Verification items for the finished model (mm, model axes). A direction names the side the tool comes from. Round coordinates to 2 decimals unless told otherwise and drop trailing zeros. Write each loop counter-clockwise with the first axis right and the second up, starting at its lowest first coordinate (ties: lowest second). Pieces come first, ordered by that corner, then holes. Notation, with made-up numbers: M 89.5,-23 L 111.5,-23 A24 cw 111.5,5 Z; hole C 39.5,63.5 d3. An arc over 180 degrees is marked long. Answer in a Markdown table with one row per item. Add a question column.
1. Sectioned sample at C-C on z = 19. Record the cut outline in (x, y).
2. Go/stop test with flat-tipped pins: pin 1 Ø1 at (x, y) = (-9.5, -0.5) entering from +Z; pin 2 Ø10 at (y, z) = (-9.5, 12) entering from +X; pin 3 Ø12 at (y, z) = (6.5, 20.5) entering from -X; pin 4 Ø5 at (x, y) = (6, -0.5) entering from -Z. Record where each tip stops, or that it passes through.
3. Draft check along Y on faces 1 (the cylindrical face through (12.932, -5.362, 35.479)), 2 (the flat face through (3, -3, 63)), 3 (the flat face through (-10, 0, 53)). Enter one of: pulls with the +Y half, pulls with the -Y half, needs draft (parallel to the pull), parting line crosses it, or undercut.
4. Sectioned sample at D-D on y = -11. Record the cut outline in (x, z), plus the area to 3 significant figures.
5. Set-up check for faces 4 (the cylindrical face through (2.93, -13.18, 37.49)), 5 (the cylindrical face through (12.932, -5.362, 6.902)), 6 (the flat face through (0, 0, 0)), 7 (the cylindrical face through (3.233, -1.341, 63.986)), 8 (the flat face through (0, 0, 77)): record each of +Z, -Z, +X, -X, +Y, -Y from which the full face is reachable in a straight line by a thin tool's end or side.
6. Material ranges on probe 1 along Z at (x, y) = (-1.75, 11.5); probe 2 along Z at (x, y) = (0.5, -2.5); probe 3 along Y at (x, z) = (10, 55.5), recorded low to high.
7. Sectioned sample at A-A on x = 0. Record the cut outline in (y, z), plus the area to 4 significant figures.
8. Sectioned sample at B-B on y = 10. Record the cut outline in (x, z), plus the area to 3 significant figures.
```python
from build123d import *

# Parameters (mm, degrees)
SKETCH1_R           = 14
BOSS_EXTRUDE1_DEPTH = 63
SKETCH2_R           = 3.5
BOSS_EXTRUDE2_DEPTH = 2
SKETCH3_R           = 2
BOSS_EXTRUDE3_DEPTH = 12
SKETCH4_R           = 14.5
BOSS_EXTRUDE4_DEPTH = 20
SKETCH5_OUTSIDE_W   = 48.448
SKETCH5_OUTSIDE_H   = 48.448
SKETCH5_OUTSIDE_R   = 13.5
CUT_EXTRUDE1_DEPTH  = 1
SKETCH6_R           = 1.75
CUT_EXTRUDE2_DEPTH  = 10


with BuildPart() as part:
    # Sketch1 → Boss-Extrude1 (new body)
    with BuildSketch(Plane.XY):
        Circle(SKETCH1_R)
    extrude(amount=BOSS_EXTRUDE1_DEPTH)

    # Sketch2 → Boss-Extrude2 (add)
    with BuildSketch(Plane.XY.offset(63)):
        Circle(SKETCH2_R)
    extrude(amount=BOSS_EXTRUDE2_DEPTH)

    # Sketch3 → Boss-Extrude3 (add)
    with BuildSketch(Plane.XY.offset(65)):
        Circle(SKETCH3_R)
    extrude(amount=BOSS_EXTRUDE3_DEPTH)

    # Sketch4 → Boss-Extrude4 (add)
    with BuildSketch(Plane(origin=(0, 0, 14), x_dir=(-1, 0, 0), z_dir=(0, 0, -1))):
        Circle(SKETCH4_R)
    extrude(amount=-BOSS_EXTRUDE4_DEPTH)

    # Sketch5 outside → Cut-Extrude1 (cut)
    with BuildSketch(Plane(origin=(0, 0, 37), x_dir=(-1, 0, 0), z_dir=(0, 0, -1))):
        Rectangle(SKETCH5_OUTSIDE_W, SKETCH5_OUTSIDE_H)
        Circle(SKETCH5_OUTSIDE_R, mode=Mode.SUBTRACT)
    extrude(amount=-CUT_EXTRUDE1_DEPTH, mode=Mode.SUBTRACT)

    # Sketch6 → Cut-Extrude2 (cut)
    with BuildSketch(Plane.XY.offset(63)):
        with Locations((-10, 0)):
            Circle(SKETCH6_R)
        with Locations((10, 0)):
            Circle(SKETCH6_R)
    extrude(amount=-CUT_EXTRUDE2_DEPTH, mode=Mode.SUBTRACT)


solid = part.part
```
Geometry check:
| question | item | result |
|---|---|---|
| 1 | outline | C 0,0 d29 |
| 2 | pin 1 | stops at z = 53 |
| 2 | pin 2 | stops at x = 13.64 |
| 2 | pin 3 | stops at x = -14.49 |
| 2 | pin 4 | stops at z = 0 |
| 3 | face 1 | parting line crosses it |
| 3 | face 2 | needs draft |
| 3 | face 3 | undercut |
| 4 | outline | M -9.45,14 L -8.66,14 L -8.66,0 L 8.66,0 L 8.66,14 L 9.45,14 L 9.45,34 L 8.66,34 L 8.66,37 L 7.83,37 L 7.83,38 L 8.66,38 L 8.66,63 L -8.66,63 L -8.66,38 L -7.83,38 L -7.83,37 L -8.66,37 L -8.66,34 L -9.45,34 Z |
| 4 | area | 1,120 mm2 |
| 5 | face 4 | none |
| 5 | face 5 | -Z |
| 5 | face 6 | -Z, +X, -X, +Y, -Y |
| 5 | face 7 | +Z |
| 5 | face 8 | +Z, +X, -X, +Y, -Y |
| 6 | probe 1 | z = 0 to 63 |
| 6 | probe 2 | z = 0 to 65 |
| 6 | probe 3 | y = -9.8 to -1.75, 1.75 to 9.8 |
| 7 | outline | M -14.5,14 L -14,14 L -14,0 L 14,0 L 14,14 L 14.5,14 L 14.5,34 L 14,34 L 14,37 L 13.5,37 L 13.5,38 L 14,38 L 14,63 L 3.5,63 L 3.5,65 L 2,65 L 2,77 L -2,77 L -2,65 L -3.5,65 L -3.5,63 L -14,63 L -14,38 L -13.5,38 L -13.5,37 L -14,37 L -14,34 L -14.5,34 Z |
| 7 | area | 1,845 mm2 |
| 8 | outline | M -10.5,14 L -9.8,14 L -9.8,0 L 9.8,0 L 9.8,14 L 10.5,14 L 10.5,34 L 9.8,34 L 9.8,37 L 9.07,37 L 9.07,38 L 9.8,38 L 9.8,63 L -9.8,63 L -9.8,38 L -9.07,38 L -9.07,37 L -9.8,37 L -9.8,34 L -10.5,34 Z |
| 8 | area | 1,260 mm2 |
